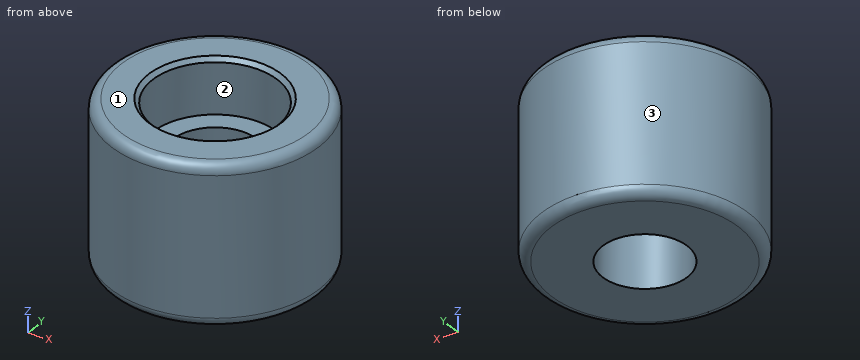
from build123d import *

# Parameters (mm, degrees)
SKETCH1_R           = 16.51
SKETCH1_R_2         = 4.7625
BOSS_EXTRUDE1_DEPTH = 25.146
FILLET2_R           = 1.5875


with BuildPart() as part:
    # Sketch1 → Boss-Extrude1 (new body)
    with BuildSketch(Plane.XY):
        with Locations((-66.414856712, -15.92976268)):
            Circle(SKETCH1_R)
        with Locations((-66.414856712, -15.92976268)):
            Circle(SKETCH1_R_2, mode=Mode.SUBTRACT)
    extrude(amount=BOSS_EXTRUDE1_DEPTH)

    # Fillet2
    fillet2_edges = [part.edges().sort_by_distance(p)[0] for p in [
        (-82.924856712, -15.92976268, 0),
        (-82.924856712, -15.92976268, 25.146),
    ]]
    fillet(fillet2_edges, radius=FILLET2_R)

    # Sketch4 → CBORE for 1/2 Socket Shoulder Screw1 (revolve, cut)
    with BuildSketch(Plane(origin=(-66.414856712, -15.92976268, 25.146), x_dir=(0, -1, 0), z_dir=(1, 0, 0))):
        Polygon((0, 0), (0, 25.146), (6.74624, 25.146), (6.74624, 8.6868), (9.92124, 8.6868), (9.92124, 0.635), (10.55624, 0), align=None)
    revolve(axis=Axis((-66.414856712, -15.92976268, 31.496), (0, 0, -1)), mode=Mode.SUBTRACT)


solid = part.part
Can you work these out from the model? Positions are in its coordinate system, mm. Face numbers are marked on the shaded views. Coordinates: 2 decimals unless noted, no trailing zeros. Loops run counter-clockwise (first coordinate to the right, second up) from the corner with the lowest first, then second, coordinate; pieces in that order, holes last. Notation, with made-up numbers: M -25,-6.75 L 31,-6.75 A29 cw 31,26.25 Z; hole C 39,75.25 d2. An arc over 180 degrees is marked long. Answer as CSV lines item,"result". Start each with the question number.
1. Suppose I cut it at B-B, the plane z = 19.75. List the corners of the cut face in (x, y) for me, plus the area to 3 significant figures.
2. If I drill on probe 1 along Z at (x, y) = (-57, -18); probe 2 along X at (y, z) = (-16, 4.5) (3 decimals); probe 3 along Y at (x, z) = (-69.5, 21.5), over which ranges is the centre line in solid material (lowest first)? Write a range as [from, to].
3. Suppose I cut it at A-A, the plane z = 14.75. List the corners of the cut face in (x, y) for me.
4. For pin 1 Ø15.5 at (x, y) = (-66.41, -15.93) entering from +Z; pin 2 Ø1 at (y, z) = (-8, 4) entering from +X; pin 3 Ø2 at (x, z) = (-70.5, 13) entering from +Y, each with a flat end and sliding along its axis, tell me the tip position at first contact or that it passes through.
5. Thinking about a two-plate mould opening in Y: for the marked faces 1, 2 and 3, which applies, +Y half, -Y half, draft (parallel to the pull), parting line (faces both ways), or undercut?
Output:
1,outline,"C -66.41,-15.93 d33.02; hole C -66.41,-15.93 d19.84"
1,area,"547 mm^2"
2,probe 1,"z = [0, 16.46]"
2,probe 2,"x = [-82.925, -73.161], [-59.669, -49.905]"
2,probe 3,"y = [-32.15, -25.36], [-6.5, 0.29]"
3,outline,"C -66.41,-15.93 d33.02; hole C -66.41,-15.93 d13.49"
4,pin 1,"stops at z = 16.46"
4,pin 2,"stops at x = -51.67"
4,pin 3,"stops at y = 0.29"
5,face 1,"draft"
5,face 2,"undercut"
5,face 3,"parting line"
